Geometry check sheet. Reference: the model listing, model coordinates, mm. Give positions to 0.01 mm unless a question says otherwise; leave off trailing zeros. Order: outer loops, then holes, each group sorted by start corner. A loop starts at its lowest first (then second) coordinate and runs counter-clockwise, first axis right, second up.
from build123d import *


with BuildPart() as part:
    # Sketch1 → Revolve1 (revolve)
    with BuildSketch(Plane.XY):
        with BuildLine():
            Line((-0.740666673, 8.5), (10.259333327, 8.5))
            ThreePointArc((10.259333327, 8.5), (10.612886718, 8.646446609), (10.759333327, 9))
            Line((10.759333327, 9), (10.759333327, 12))
            Line((10.759333327, 12), (7.20882307, 12))
            ThreePointArc((7.20882307, 12), (4.759333327, 11), (2.309843584, 12))
            Line((2.309843584, 12), (-1.240666673, 12))
            Line((-1.240666673, 12), (-1.240666673, 9))
            ThreePointArc((-1.240666673, 9), (-1.094220063, 8.646446609), (-0.740666673, 8.5))
        make_face()
    revolve(axis=Axis((-52.659695599, 0, 0), (1, 0, 0)))


solid = part.part
Item 1: Sectioned sample at A-A (y = 0). Enter the section's corners in (x, z).
Reported:
outline: (-1.24, -12) - (2.31, -12) arc R3.5 cw to (7.21, -12) - (10.76, -12) - (10.76, -9) arc R0.5 ccw to (10.26, -8.5) - (-0.74, -8.5) arc R0.5 ccw to (-1.24, -9) - close; (-1.24, 9) arc R0.5 ccw to (-0.74, 8.5) - (10.26, 8.5) arc R0.5 ccw to (10.76, 9) - (10.76, 12) - (7.21, 12) arc R3.5 cw to (2.31, 12) - (-1.24, 12) - close
Item 2: Sectioned sample at B-B (x = 6.75). Enter the section's corners in (y, z).
Reported:
outline: circle Ø23.24 at (0, 0); hole circle Ø17 at (0, 0)
Item 3: Scan lines: L1, parallel to Z at x = 4.25, y = 0; L2, parallel to Y at x = 7.75, z = 3.5; L3, parallel to Y at x = 8, z = 2. Record each from-to range of solid material in increasing order.
Reported:
L1: z = -11.04 to -8.5, 8.5 to 11.04
L2: y = -11.48 to -7.75, 7.75 to 11.48
L3: y = -11.83 to -8.26, 8.26 to 11.83
Item 4: Gauge pin test, flat ends, axial feed: pin 1 (8 mm diameter, centred on y = 2.5, z = -3.5, fed in from -X); pin 2 (4 mm diameter, centred on x = 8, y = -6, fed in from +Z); pin 3 (5 mm diameter, centred on x = 3, z = 5, fed in from +Y); pin 4 (1 mm diameter, centred on x = 3, z = -3, fed in from -Y). Record the tip position at first contact, or that the pin passes through.
Reported:
pin 1: passes through
pin 2: stops at z = 11.31
pin 3: stops at y = 11.72
pin 4: stops at y = -11.46
Item 5: Sectioned sample at C-C (x = 4.75). Enter the section's corners in (y, z).
Reported:
outline: circle Ø22 at (0, 0); hole circle Ø17 at (0, 0)
Item 6: Draft check along Y on faces 1 (the cylindrical face through (0.51, -11.99, 0.53)), 2 (the flat face through (-1.241, 2, 9)), 3 (the cylindrical face through (4.836, 4.57, 7.167)). Enter one of: released by +Y, released by -Y, zero draft, split by the parting line, or undercut.
Reported:
face 1: split by the parting line
face 2: zero draft
face 3: undercut
